Could you check a few things on this model? Use its own coordinates, in mm. Face numbers are marked on the shaded views. A direction names the side the tool comes from. Coordinates: 2 decimals unless noted, no trailing zeros. Order: outer loops, then holes, each group sorted by start corner. A loop starts at its lowest first (then second) coordinate and runs counter-clockwise, first axis right, second up. Notation, with made-up numbers: (-5, -14) -> (31, -14) arc R31 ccw to (31, 10) -> close; hole circle Ø8 at (86, 58). An arc over 180 degrees is marked (long way). Use a Markdown table: item, result. Add a question column.
1) Which directions (+Z, -Z, +X, -X, +Y, -Y) give clear straight access to the entire face, cutting with the end or side of a thin tool? Please do the marked faces 1 and 2.
2) Will these pins go through, and if not, where does the flat tip stop? pin 1 Ø1.5 at (y, z) = (1, -2) entering from -X; pin 2 Ø1.5 at (x, z) = (3, 0) entering from -Y; pin 3 Ø0.8 at (x, y) = (0, 2.5) entering from -Z; pin 4 Ø0.5 at (x, y) = (0.5, 2.5) entering from +Z.
3) Thinking about a two-plate mould opening in X: for the marked faces 3, 4, 5 and 6, which applies, +X half, -X half, draft (parallel to the pull), parting line (faces both ways), or undercut?
4) If we section it at A-A (y = -1.15): Write out the boundary of the cut face in (x, z).
5) If I drill on L1, parallel to Z at x = 0, y = 2.75; L2, parallel to X at y = -0.9, z = 0; L3, parallel to Z at x = -0.5, y = 2.55, over which ranges is the centre line in solid material (lowest first)? Write a range as [from, to].
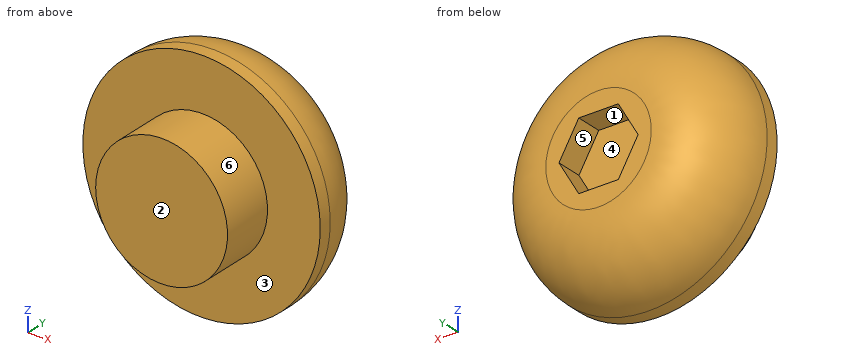
```python
from build123d import *

# Parameters (mm, degrees)
SKETCH1_R           = 4.5
BOSS_EXTRUDE1_DEPTH = 3
FILLET1_R           = 2.5
CUT_EXTRUDE1_DEPTH  = 1
SKETCH3_R           = 2.5
BOSS_EXTRUDE2_DEPTH = 2


with BuildPart() as part:
    # Sketch1 → Boss-Extrude1 (new body)
    with BuildSketch(Plane(origin=(0, 0, 0), x_dir=(1, 0, 0), z_dir=(0, 1, 0))):
        Circle(SKETCH1_R)
    extrude(amount=BOSS_EXTRUDE1_DEPTH)

    # Fillet1
    fillet1_edges = [part.edges().sort_by_distance(p)[0] for p in [
        (-4.5, 3, 0),
    ]]
    fillet(fillet1_edges, radius=FILLET1_R)

    # Sketch2 → Cut-Extrude1 (cut)
    with BuildSketch(Plane(origin=(0, 3, 0), x_dir=(1, 0, 0), z_dir=(0, 1, 0))):
        Polygon((1.5, 0), (0.75, 1.299038106), (-0.75, 1.299038106), (-1.5, 0), (-0.75, -1.299038106), (0.75, -1.299038106), align=None)
    extrude(amount=-CUT_EXTRUDE1_DEPTH, mode=Mode.SUBTRACT)

    # Sketch3 → Boss-Extrude2 (add)
    with BuildSketch(Plane(origin=(0, 0, 0), x_dir=(-1, 0, 0), z_dir=(0, -1, 0))):
        Circle(SKETCH3_R)
    extrude(amount=BOSS_EXTRUDE2_DEPTH)


solid = part.part
```
Answer sheet:
| question | item | result |
|---|---|---|
| 1 | face 1 | +Y |
| 1 | face 2 | +Z, -Z, +X, -X, -Y |
| 2 | pin 1 | x = -4.3 |
| 2 | pin 2 | y = -2 |
| 2 | pin 3 | z = -3.92 |
| 2 | pin 4 | z = 3.75 |
| 3 | face 3 | draft |
| 3 | face 4 | undercut |
| 3 | face 5 | undercut |
| 3 | face 6 | parting line |
| 4 | outline | circle Ø5 at (0, 0) |
| 5 | L1 | [-3.09, -1.3], [1.3, 3.09] |
| 5 | L2 | [-2.5, 2.5] |
| 5 | L3 | [-3.39, -1.3], [1.3, 3.39] |
